Model file for the job. Use its own axes, mm. Face numbers are marked on the shaded views. A direction names the side the tool comes from. Round coordinates to 2 decimals unless told otherwise and drop trailing zeros. Loops run counter-clockwise (first coordinate to the right, second up) from the corner with the lowest first, then second, coordinate; pieces in that order, holes last. Notation, with made-up numbers: M 1.5,16 L 39.5,16 A23 cw 39.5,35 Z; hole C 82,-11 d11. An arc over 180 degrees is marked long. Use a Markdown table: item, result. Add a question column.
Q1. Cut at C-C (x = 8). Give the cut face in (y, z).
Q2. Probe line 1 (Z direction, x = 123.5, y = -15); line 2 (X direction, y = -3, z = -61); line 3 (Y direction, x = 7.05, z = -41.25). List the from-to ranges inside material, lowest first. Write a range as from..to.
Q3. Cut at D-D (y = -15). Give the cut face in (x, z), plus the area to 3 significant figures.
Q4. Cut at B-B (x = 95.5). Give the cut face in (y, z), plus the area to 3 significant figures.
Q5. Mould opens along Z. For the marked faces 1 and 2 say: +Z half, -Z half, draft (parallel to the pull), parting line (faces both ways), or undercut.
Q6. Tool access for the marked faces 3 and 4: list every direction of +Z, -Z, +X, -X, +Y, -Y with a clear straight run to the whole face (end or side of a thin tool).
Q7. Pin check, flat tips, straight feed: pin 1 (3 mm diameter, centred on x = 46.5, y = 7, fed in from +Z); pin 2 (4 mm diameter, centred on y = -18, z = -50.5, fed in from +X); pin 3 (3 mm diameter, centred on y = 6.5, z = -37.5, fed in from -X). Stop position of each tip, or through.
Q8. Cut at A-A (y = 3.5). Give the cut face in (x, z).
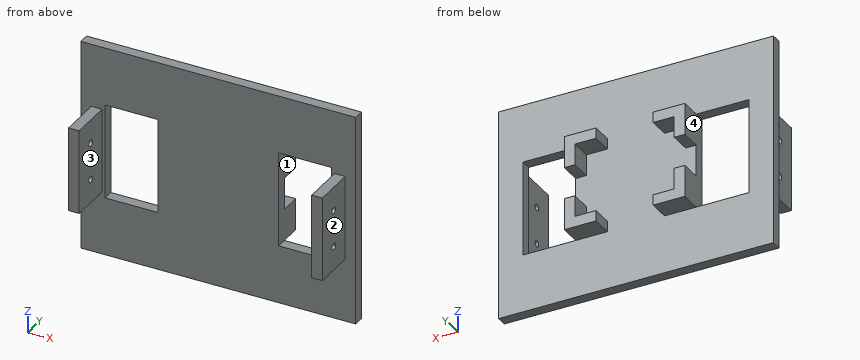
Autodesk Inventor part; units mm, degrees
ref_plane "YZ Plane" through (0, 0, 0) normal (1, 0, 0) x (0, 1, 0)
ref_plane "XZ Plane" through (0, 0, 0) normal (0, 1, 0) x (-1, 0, 0)
ref_plane "XY Plane" through (0, 0, 0) normal (0, 0, 1) x (1, 0, 0)
sketch "Sketch1" plane through (0, 0, 0) normal (0, 1, 0) x (-1, 0, 0)
  line L0 (0, 0) -> (-130, 0)
  line L1 (-130, 0) -> (-130, -100)
  line L2 (-130, -100) -> (0, -100)
  line L3 (0, -100) -> (0, 0)
  line L4 (-41.5, -67.5) -> (-88.5, -67.5) construction
  line L5 (-88.5, -67.5) -> (-88.5, -32.5) construction
  line L6 (-88.5, -32.5) -> (-41.5, -32.5) construction
  line L7 (-41.5, -32.5) -> (-41.5, -67.5) construction
  line L8 (-41.5, -50) -> (-88.5, -50) construction
  line L9 (-65, -67.5) -> (-65, -32.5) construction
  line L10 (-41.5, -32.5) -> (-41.5, -42.5)
  line L11 (-36.5, -42.5) -> (-41.5, -42.5)
  line L12 (-36.5, -42.5) -> (-36.5, -27.5)
  line L13 (-36.5, -27.5) -> (-51.5, -27.5)
  line L14 (-51.5, -27.5) -> (-51.5, -32.5)
  line L15 (-51.5, -32.5) -> (-41.5, -32.5)
  line L16 (-93.5, -42.5) -> (-88.5, -42.5)
  line L17 (-93.5, -42.5) -> (-93.5, -27.5)
  line L18 (-93.5, -27.5) -> (-78.5, -27.5)
  line L19 (-78.5, -27.5) -> (-78.5, -32.5)
  line L20 (-78.5, -32.5) -> (-88.5, -32.5)
  line L21 (-88.5, -42.5) -> (-88.5, -32.5)
  line L22 (-36.5, -57.5) -> (-41.5, -57.5)
  line L23 (-36.5, -57.5) -> (-36.5, -72.5)
  line L24 (-36.5, -72.5) -> (-51.5, -72.5)
  line L25 (-51.5, -72.5) -> (-51.5, -67.5)
  line L26 (-93.5, -57.5) -> (-88.5, -57.5)
  line L27 (-93.5, -57.5) -> (-93.5, -72.5)
  line L28 (-93.5, -72.5) -> (-78.5, -72.5)
  line L29 (-78.5, -72.5) -> (-78.5, -67.5)
  line L30 (-41.5, -57.5) -> (-41.5, -67.5)
  line L31 (-51.5, -67.5) -> (-41.5, -67.5)
  line L32 (-78.5, -67.5) -> (-88.5, -67.5)
  line L33 (-88.5, -57.5) -> (-88.5, -67.5)
  line L34 (-11.5, -72.5) -> (-36.5, -72.5)
  line L35 (-36.5, -72.5) -> (-36.5, -27.5)
  line L36 (-36.5, -27.5) -> (-11.5, -27.5)
  line L37 (-11.5, -27.5) -> (-11.5, -72.5)
  line L38 (-118.5, -72.5) -> (-93.5, -72.5)
  line L39 (-93.5, -72.5) -> (-93.5, -27.5)
  line L40 (-93.5, -27.5) -> (-118.5, -27.5)
  line L41 (-118.5, -27.5) -> (-118.5, -72.5)
  point P0 (0, -50)
  point P1 (-65, -100)
  point P2 (-24, -72.5)
  point P3 (-24, -57.5)
  point P4 (-24, -27.5)
  dimension "d0" = 130
  dimension "d1" = 100
  dimension "d4" = 47
  dimension "d5" = 35
  dimension "d6" = 5
  dimension "d7" = 5
  dimension "d8" = 10
  dimension "d9" = 10
  dimension "d26" = 25
  dimension "d27" = 0
extrude "Extrusion1" add sketch "Sketch1" against normal blind 5 contours L3 L2 L1 L0 | L15 L14 L13 L12 L11 L10 | L23 L24 L25 L31 L30 L22 | L17 L18 L19 L20 L21 L16 | L26 L33 L32 L29 L28 L27
extrude "Extrusion2" add sketch "Sketch1" along normal blind 10 contours L15 L14 L13 L12 L11 L10 | L23 L24 L25 L31 L30 L22 | L17 L18 L19 L20 L21 L16 | L26 L33 L32 L29 L28 L27
sketch "Sketch2" plane through (0, -5, 0) normal (0, -1, 0) x (1, 0, 0)
  line L0 (120, -30) -> (125, -30)
  line L1 (125, -30) -> (125, -70)
  line L2 (125, -70) -> (120, -70)
  line L3 (120, -70) -> (120, -30)
  line L4 (130, -100) -> (130, 0)
  line L5 (0, 0) -> (130, 0)
  line L6 (65, 0) -> (65, -100) construction
  line L7 (130, -100) -> (0, -100)
  line L8 (10, -30) -> (5, -30)
  line L9 (5, -30) -> (5, -70)
  line L10 (5, -70) -> (10, -70)
  line L11 (10, -70) -> (10, -30)
  point P0 (125, -50)
  point P1 (130, -50)
  dimension "d12" = 5
  dimension "d13" = 40
  dimension "d14" = 5
extrude "Extrusion3" add sketch "Sketch2" along normal blind 20
sketch "Sketch3" plane through (5, -5, -70) normal (-1, 0, 0) x (0, 0, 1)
  line L0 (11.25, -10) -> (28.75, -10) construction
  line L1 (70, 0) -> (-30, 0)
  point P0 (70, 5)
  point P1 (20, 0)
  point P2 (20, -10)
  dimension "d17" = 17.5
  dimension "d18" = 10
hole "Hole1" at (5, -15, -41.25) at (5, -15, -58.75) direction (1, 0, 0) diameter 3.1 end through all
properties part number "Chasis 3"
Checked values:
| question | item | result |
|---|---|---|
| 1 | outline | M -25,-70 L -5,-70 L -5,-100 L 0,-100 L 0,0 L -5,0 L -5,-30 L -25,-30 Z; hole C -15,-58.75 d3.1; hole C -15,-41.25 d3.1 |
| 2 | line 1 | z = -70..-60.3, -57.2..-42.8, -39.7..-30 |
| 2 | line 2 | x = 0..11.5, 36.5..93.5, 118.5..130 |
| 2 | line 3 | y = -25..-16.55, -13.45..0 |
| 3 | outline | M 5,-70 L 10,-70 L 10,-60.3 L 5,-60.3 Z; M 5,-57.2 L 10,-57.2 L 10,-42.8 L 5,-42.8 Z; M 5,-39.7 L 10,-39.7 L 10,-30 L 5,-30 Z; M 120,-70 L 125,-70 L 125,-60.3 L 120,-60.3 Z; M 120,-57.2 L 125,-57.2 L 125,-42.8 L 120,-42.8 Z; M 120,-39.7 L 125,-39.7 L 125,-30 L 120,-30 Z |
| 3 | area | 338 mm^2 |
| 4 | outline | M -5,-100 L 0,-100 L 0,-72.5 L -5,-72.5 Z; M -5,-27.5 L 0,-27.5 L 0,0 L -5,0 Z |
| 4 | area | 275 mm^2 |
| 5 | face 1 | undercut |
| 5 | face 2 | draft |
| 6 | face 3 | +Z, -Z, -Y |
| 6 | face 4 | +Y, -Y |
| 7 | pin 1 | stops at z = -27.5 |
| 7 | pin 2 | stops at x = 125 |
| 7 | pin 3 | stops at x = 36.5 |
| 8 | outline | M 36.5,-72.5 L 51.5,-72.5 L 51.5,-67.5 L 41.5,-67.5 L 41.5,-57.5 L 36.5,-57.5 Z; M 36.5,-42.5 L 41.5,-42.5 L 41.5,-32.5 L 51.5,-32.5 L 51.5,-27.5 L 36.5,-27.5 Z; M 78.5,-72.5 L 93.5,-72.5 L 93.5,-57.5 L 88.5,-57.5 L 88.5,-67.5 L 78.5,-67.5 Z; M 78.5,-32.5 L 88.5,-32.5 L 88.5,-42.5 L 93.5,-42.5 L 93.5,-27.5 L 78.5,-27.5 Z |
